Read the model definition and answer for the solid it produces. Units are mm, in the model's axes. Give positions to 0.01 mm unless a question says otherwise; leave off trailing zeros. Write each loop counter-clockwise with the first axis right and the second up, starting at its lowest first coordinate (ties: lowest second). Pieces come first, ordered by that corner, then holes. Notation, with made-up numbers: (45, -3.75) -> (61, -3.75) arc R11 ccw to (61, 6.25) -> close; hole circle Ø4 at (33, 62). An arc over 180 degrees is marked (long way). Answer as CSV lines item,"result". Start each with the question number.
1. The part is cut by section A-A, the plane z = 8.5. Determine the outline of the cut face in (x, y), and give its area (3 significant figures).
2. Given pin 1 (3.5 mm diameter, centred on x = -483, z = 1.5, fed in from +Y); pin 2 (1 mm diameter, centred on x = -310.5, y = -10, fed in from +Z), each flat-ended and moving along its own axis, determine where each tip first touches the part or whether it passes through.
3. Find the intervals of material crossed by line 1 (X direction, y = -12.5, z = 1.9); line 2 (Y direction, x = 155, z = 5.5); line 3 (Y direction, x = -335, z = 1.3), in increasing order.
4. The part is cut by section B-B, the plane x = 233. Determine the outline of the cut face in (y, z), and give its area (3 significant figures).
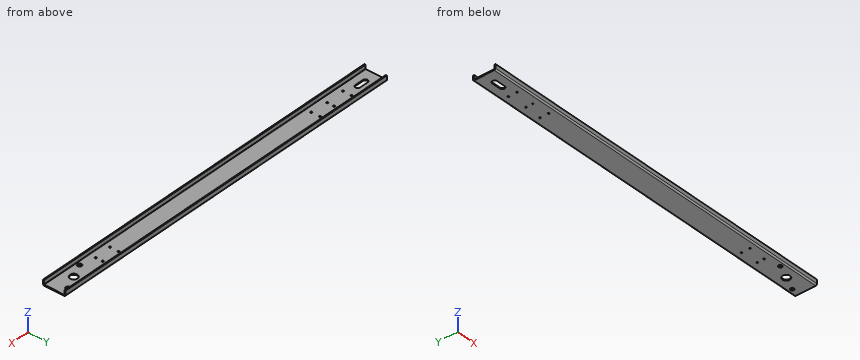
from build123d import *

# Parameters (mm, degrees)
BASE_FLANGE1_DEPTH          = 535
CUT_EXTRUDE1_DEPTH          = 537.120555472
M5_TAPPED_HOLE1_D           = 4.2
M5_TAPPED_HOLE1_CSINK_D     = 5.05
M5_TAPPED_HOLE1_CSINK_ANGLE = 90
M5_TAPPED_HOLE2_D           = 4.2
M5_TAPPED_HOLE2_CSINK_D     = 5.05
M5_TAPPED_HOLE2_CSINK_ANGLE = 90
M5_TAPPED_HOLE3_D           = 4.2
M5_TAPPED_HOLE3_CSINK_D     = 5.05
M5_TAPPED_HOLE3_CSINK_ANGLE = 90
SKETCH16_R                  = 11
CUT_EXTRUDE2_DEPTH          = 537.120555472
M12_TAPPED_HOLE1_AT_2_COUNT = 2
M12_TAPPED_HOLE1_AT_2_PITCH = 90


# Sheet-metal steps are written as plain solids
with BuildPart() as part:
    # Sketch1 → Base-Flange1 (new, symmetric)
    with BuildSketch(Plane(origin=(0, 0, 0), x_dir=(0, 0, -1), z_dir=(1, 0, 0))):
        with BuildLine():
            Line((-15, -32.5), (-3.7366, -32.5))
            ThreePointArc((-3.7366, -32.5), (-1.094424801, -31.405575199), (0, -28.7634))
            Line((0, -28.7634), (0, 28.7634))
            ThreePointArc((0, 28.7634), (-1.094424801, 31.405575199), (-3.7366, 32.5))
            Line((-3.7366, 32.5), (-15, 32.5))
            Line((-15, 32.5), (-15, 29.5))
            Line((-15, 29.5), (-3.7366, 29.5))
            ThreePointArc((-3.7366, 29.5), (-3.215745145, 29.284254855), (-3, 28.7634))
            Line((-3, 28.7634), (-3, -28.7634))
            ThreePointArc((-3, -28.7634), (-3.215745145, -29.284254855), (-3.7366, -29.5))
            Line((-3.7366, -29.5), (-15, -29.5))
            Line((-15, -29.5), (-15, -32.5))
        make_face()
    extrude(amount=BASE_FLANGE1_DEPTH, both=True)

    # Sketch6 → Cut-Extrude1 (cut, through all)
    with BuildSketch(Plane.XY.offset(3)):
        with BuildLine():
            Line((-500, 7), (-475, 7))
            ThreePointArc((-475, 7), (-468, 0), (-475, -7))
            Line((-475, -7), (-500, -7))
            ThreePointArc((-500, -7), (-507, 0), (-500, 7))
        make_face()
    extrude(amount=-CUT_EXTRUDE1_DEPTH, mode=Mode.SUBTRACT)

    # M5 Tapped Hole1 (through all)
    with Locations(Plane.XY.offset(3)):
        with Locations((-440, 12.5), (-440, -12.5)):
            CounterSinkHole(M5_TAPPED_HOLE1_D / 2, M5_TAPPED_HOLE1_CSINK_D / 2, counter_sink_angle=M5_TAPPED_HOLE1_CSINK_ANGLE)

    # M5 Tapped Hole2 (through all)
    with Locations(Plane.XY.offset(3)):
        with Locations((-385, 10), (-385, -10)):
            m5_tapped_hole2 = CounterSinkHole(M5_TAPPED_HOLE2_D / 2, M5_TAPPED_HOLE2_CSINK_D / 2, counter_sink_angle=M5_TAPPED_HOLE2_CSINK_ANGLE)

    # M5 Tapped Hole3 (through all)
    with Locations(Plane.XY.offset(3)):
        with Locations((-335, 12.5), (-335, -12.5)):
            m5_tapped_hole3 = CounterSinkHole(M5_TAPPED_HOLE3_D / 2, M5_TAPPED_HOLE3_CSINK_D / 2, counter_sink_angle=M5_TAPPED_HOLE3_CSINK_ANGLE)

    # Mirror1: M5 Tapped Hole2, M5 Tapped Hole3 across plane
    add(m5_tapped_hole2.mirror(Plane(origin=(0, 0, 0), x_dir=(0, 0, 1), z_dir=(1, 0, 0))), mode=Mode.SUBTRACT)
    add(m5_tapped_hole3.mirror(Plane(origin=(0, 0, 0), x_dir=(0, 0, 1), z_dir=(1, 0, 0))), mode=Mode.SUBTRACT)

    # Sketch16 → Cut-Extrude2 (cut, through all)
    with BuildSketch(Plane.XY.offset(3)):
        with Locations((470, 0)):
            Circle(SKETCH16_R)
    extrude(amount=-CUT_EXTRUDE2_DEPTH, mode=Mode.SUBTRACT)

    # Sketch20 → M12 Tapped Hole1 (revolve, cut)
    with BuildSketch(Plane(origin=(428.977162095, -18.496669166, 3), x_dir=(0, -1, 0), z_dir=(1, 0, 0))):
        Polygon((0, 0), (0, 3), (5.1, 3), (5.1, 0.925), (6.025, 0), align=None)
    m12_tapped_hole1 = revolve(axis=Axis((428.977162095, -18.496669166, 9.35), (0, 0, -1)), mode=Mode.SUBTRACT)

    # M12 Tapped Hole1 at 2: M12 Tapped Hole1 ×2
    with Locations(*[Vector(0.9116186201067192, 0.4110370925776907, 0) * (i * M12_TAPPED_HOLE1_AT_2_PITCH) for i in range(1, M12_TAPPED_HOLE1_AT_2_COUNT)]):
        add(m12_tapped_hole1, mode=Mode.SUBTRACT)


solid = part.part
Results found:
1,outline,"(-535, -32.5) -> (535, -32.5) -> (535, -29.5) -> (-535, -29.5) -> close; (-535, 29.5) -> (535, 29.5) -> (535, 32.5) -> (-535, 32.5) -> close"
1,area,"6,420 mm²"
2,pin 1,"stops at y = 32.47"
2,pin 2,"stops at z = 3"
3,line 1,"x = -535 to -442.1, -437.9 to -337.1, -332.9 to 332.9, 337.1 to 535"
3,line 2,"y = -32.5 to -29.5, 29.5 to 32.5"
3,line 3,"y = -31.6 to -14.6, -10.4 to 10.4, 14.6 to 31.6"
4,outline,"(-32.5, 3.74) arc R3.74 ccw to (-28.76, 0) -> (28.76, 0) arc R3.74 ccw to (32.5, 3.74) -> (32.5, 15) -> (29.5, 15) -> (29.5, 3.74) arc R0.74 cw to (28.76, 3) -> (-28.76, 3) arc R0.74 cw to (-29.5, 3.74) -> (-29.5, 15) -> (-32.5, 15) -> close"
4,area,"261 mm²"
